from build123d import *

# Parameters (mm, degrees)
BOSS_EXTRUDE1_DEPTH = 3
SKETCH2_R           = 30.5
CUT_EXTRUDE1_DEPTH  = 50.876169719
SKETCH3_W           = 2
SKETCH3_H           = 2
BOSS_EXTRUDE2_DEPTH = 3
SKETCH4_W           = 2
SKETCH4_H           = 2
BOSS_EXTRUDE3_DEPTH = 3


with BuildPart() as part:
    # Sketch1 → Boss-Extrude1 (new body)
    with BuildSketch(Plane(origin=(0, 0, 0), x_dir=(1, 0, 0), z_dir=(0, 1, 0))):
        Polygon((-32.718400228, 18.380414028), (-32.277105594, -19.144758755), (0.441294634, -37.525172783), (32.718400228, -18.380414028), (32.277105594, 19.144758755), (-0.441294634, 37.525172783), align=None)
    extrude(amount=BOSS_EXTRUDE1_DEPTH)

    # Sketch2 → Cut-Extrude1 (cut, through all)
    with BuildSketch(Plane(origin=(0, 3, 0), x_dir=(1, 0, 0), z_dir=(0, 1, 0))):
        with Locations(Location((0, 0, 0), (0, 0, 270))):
            Circle(SKETCH2_R)
    extrude(amount=-CUT_EXTRUDE1_DEPTH, mode=Mode.SUBTRACT)

    # Sketch3 → Boss-Extrude2 (add)
    with BuildSketch(Plane(origin=(0, 3, 0), x_dir=(1, 0, 0), z_dir=(0, 1, 0))):
        with Locations((-0.441294634, 34.010990071)):
            Rectangle(SKETCH3_W, SKETCH3_H)
    extrude(amount=BOSS_EXTRUDE2_DEPTH)

    # Sketch4 → Boss-Extrude3 (add)
    with BuildSketch(Plane(origin=(0, 3, 0), x_dir=(1, 0, 0), z_dir=(0, 1, 0))):
        with Locations((0.441294634, -34.010990071)):
            Rectangle(SKETCH4_W, SKETCH4_H)
    extrude(amount=BOSS_EXTRUDE3_DEPTH)


solid = part.part
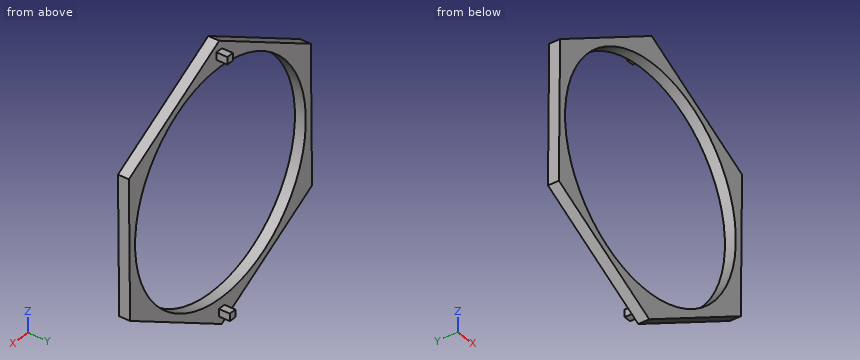
Can you work these out from the model? Positions are in its coordinate system, mm. Give positions to 0.01 mm unless a question says otherwise; leave off trailing zeros. Write each loop counter-clockwise with the first axis right and the second up, starting at its lowest first coordinate (ties: lowest second). Pieces come first, ordered by that corner, then holes. Notation, with made-up numbers: (82, -19.5) -> (107, -19.5) arc R35 cw to (107, 17.5) -> close; hole circle Ø6 at (61.25, 7). An arc over 180 degrees is marked (long way). Answer as a JSON object with one key per item and string values. Group by question number.
Item 1: Please list where these lines run through material, in increasing order: line 1 (X direction, y = 2.15, z = 0); line 2 (X direction, y = 0.95, z = -27); line 3 (Z direction, x = 26, y = 1.55). Write a range as [from, to].
Item 2: I'm going to push flat-ended pins straight in: P1, Ø19.5, axis at x = 5.5, z = -18.5, coming from the +Y side; P2, Ø2, axis at x = -1, y = 4.5, coming from the -Z side; P3, Ø1.6, axis at x = 1, y = 4, coming from the +Z side; P4, Ø1, axis at y = 1, z = 19.5, coming from the +X side. Where does each tip first touch, or does it pass through?
Item 3: Suppose I cut it at A-A (x = -25.5). Please give me the cut outline in (y, z).
Item 4: Suppose I cut it at C-C (z = 0). Please give me the cut outline in (x, y), plus the area to 3 significant figures.
Item 5: Suppose I cut it at B-B (y = 1.95). Please give me the cut outline in (x, z), plus the area to 3 significant figures.
Findings:
{
 "1": {"line 1": "x = [-32.5, -30.5], [30.5, 32.5]", "line 2": "x = [-18.19, -14.19], [14.19, 18.29]", "line 3": "z = [-22.67, -15.95], [15.95, 22.37]"},
 "2": {"P1": "passes through", "P2": "stops at z = -35.01", "P3": "stops at z = 35.01", "P4": "stops at x = 31.67"},
 "3": {"outline": "(0, -22.66) -> (3, -22.66) -> (3, -16.73) -> (0, -16.73) -> close; (0, 16.73) -> (3, 16.73) -> (3, 22.95) -> (0, 22.95) -> close"},
 "4": {"outline": "(-32.5, 0) -> (-30.5, 0) -> (-30.5, 3) -> (-32.5, 3) -> close; (30.5, 0) -> (32.5, 0) -> (32.5, 3) -> (30.5, 3) -> close", "area": "12.0 mm²"},
 "5": {"outline": "(-32.72, -18.38) -> (-0.44, -37.53) -> (32.28, -19.14) -> (32.72, 18.38) -> (0.44, 37.53) -> (-32.28, 19.14) -> close; hole circle Ø61 at (0, 0)", "area": "736 mm²"}
}
